Part model, mm, in its own coordinate system. Face numbers are marked on the shaded views. A direction names the side the tool comes from. Coordinates: 2 decimals unless noted, no trailing zeros. Loops run counter-clockwise (first coordinate to the right, second up) from the corner with the lowest first, then second, coordinate; pieces in that order, holes last. Notation, with made-up numbers: (61, 69) -> (86, 69) arc R27 cw to (86, 87) -> close; hole circle Ø9 at (-21, 43.5). An arc over 180 degrees is marked (long way). Use one line per item in the form item = value. Start each with the question number.
(1) Mould opens along X. For the marked faces 3, 4, 5 and 6 say: +X half, -X half, draft (parallel to the pull), parting line (faces both ways), or undercut.
(2) Pin check, flat tips, straight feed: P1, Ø1.8, axis at x = -3, y = 1.5, coming from the +Z side; P2, Ø1.5, axis at x = -0.5, y = 0.5, coming from the -Z side. Stop position of each tip, or through.
(3) Band-saw the part on C-C on x = 0. Give the cut face in (y, z), then the cut area to 4 significant figures.
(4) 3-axis set-ups, long thin cutter, end or side, ignore diameter. For the marked faces 1 and 2: which of +Z, -Z, +X, -X, +Y, -Y reach the whole face in a straight line?
(5) Drill centre lines: L1, parallel to Z at x = -1.25, y = -6; L2, parallel to Z at x = 1, y = -2.5; L3, parallel to Y at x = 0, z = -1.25. Where is each one in solid material? Low to high. Write a range as [from, to].
(6) Band-saw the part on A-A on z = 1.25. Give the cut face in (x, y).
(7) Band-saw the part on D-D on z = -1.15. Give the cut face in (x, y), then the cut area to 3 significant figures.
(8) Band-saw the part on B-B on y = 0. Give the cut face in (x, z), then the cut area to 4 significant figures.
Autodesk Inventor part; units mm, degrees
ref_plane "YZ Plane" through (0, 0, 0) normal (1, 0, 0) x (0, 1, 0)
ref_plane "XZ Plane" through (0, 0, 0) normal (0, 1, 0) x (-1, 0, 0)
ref_plane "XY Plane" through (0, 0, 0) normal (0, 0, 1) x (1, 0, 0)
sketch "スケッチ1" plane through (0, 0, 0) normal (0, 0, 1) x (1, 0, 0)
  line L0 (-4.5, 7) -> (4.5, 7)
  line L1 (4.5, 7) -> (4.5, -7)
  line L2 (4.5, -7) -> (-4.5, -7)
  line L3 (-4.5, -7) -> (-4.5, 7)
  line L4 (0, -9.8) -> (0, 9.8)
  line L5 (-6.3, 0) -> (6.3, 0)
  point P0 (0, 0)
  dimension "d0" = 9
  dimension "d1" = 14
extrude "押し出し1" add sketch "スケッチ1" along normal mid plane 3
sketch "スケッチ2" plane through (0, 0, 1.5) normal (0, 0, 1) x (1, 0, 0)
  line L0 (-4.5, 7) -> (-4.5, -7)
  line L1 (-4.5, 5.05) -> (1.6, 5.05)
  line L2 (1.6, 5.05) -> (1.6, -5.05)
  line L3 (1.6, -5.05) -> (-4.5, -5.05)
  line L4 (-4.5, -5.05) -> (-4.5, 5.05)
  line L5 (-6.3, 0) -> (6.3, 0)
  point P0 (0, 0)
  dimension "d4" = 6.1
  dimension "d5" = 10.1
extrude "押し出し2" cut sketch "スケッチ2" against normal blind 0.5
sketch "スケッチ3" plane through (0, 0, -1.5) normal (0, 0, -1) x (-1, 0, 0)
  circle A0 centre (0, 0) radius 1.5
  dimension "d8" = 3
extrude "押し出し3" cut sketch "スケッチ3" against normal blind 0.5
chamfer "面取り1" distance 2 angle 45 2 edges at (0, -7, -1.5) (0, 7, -1.5)
chamfer "面取り2" distance 1 angle 45 1 edges at (4.5, 0, -1.5)
properties part number "magnet_holder_ver.1"
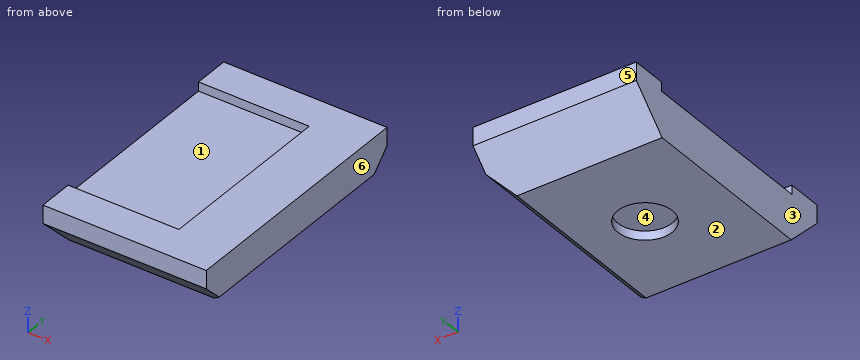
A:
q1.face_3 = -X half
q1.face_4 = undercut
q1.face_5 = draft
q1.face_6 = +X half
q2.P1 = 1
q2.P2 = -1
q3.outline = (-7, 0.5) -> (-5, -1.5) -> (-1.5, -1.5) -> (-1.5, -1) -> (1.5, -1) -> (1.5, -1.5) -> (5, -1.5) -> (7, 0.5) -> (7, 1.5) -> (5.05, 1.5) -> (5.05, 1) -> (-5.05, 1) -> (-5.05, 1.5) -> (-7, 1.5) -> close
q3.area = 31.45 mm²
q4.face_1 = +Z, -X
q4.face_2 = -Z, +X, -X, +Y, -Y
q5.L1 = [-0.5, 1.5]
q5.L2 = [-1.5, 1]
q5.L3 = [-5.25, -1.5], [1.5, 5.25]
q6.outline = (-4.5, -7) -> (4.5, -7) -> (4.5, 7) -> (-4.5, 7) -> (-4.5, 5.05) -> (1.6, 5.05) -> (1.6, -5.05) -> (-4.5, -5.05) -> close
q7.outline = (-4.5, -5.35) -> (3.85, -5.35) -> (3.85, 5.35) -> (-4.5, 5.35) -> close; hole circle Ø3 at (0, 0)
q7.area = 82.3 mm²
q8.outline = (-4.5, -1.5) -> (-1.5, -1.5) -> (-1.5, -1) -> (1.5, -1) -> (1.5, -1.5) -> (3.5, -1.5) -> (4.5, -0.5) -> (4.5, 1.5) -> (1.6, 1.5) -> (1.6, 1) -> (-4.5, 1) -> close
q8.area = 21.95 mm²
